Can you work these out from the model? Positions are in its coordinate system, mm. Face numbers are marked on the shaded views. A direction names the side the tool comes from. Coordinates: 2 decimals unless noted, no trailing zeros. Loops run counter-clockwise (first coordinate to the right, second up) from the corner with the lowest first, then second, coordinate; pieces in that order, holes last.
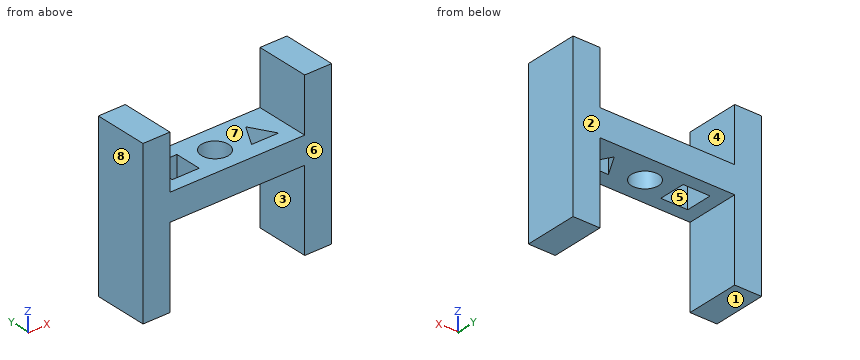
```python
from build123d import *

# Parameters (mm, degrees)
F1_DEPTH = 25.4
F2_W     = 12.7
F2_H     = 12.7
F3_DEPTH = 25.4
F4_R     = 6.35
F5_DEPTH = 25.4
F7_DEPTH = 25.4


with BuildPart() as f1:
    # F0 (on Front) → F1 (new body)
    with BuildSketch(Plane.XZ):
        Polygon((-46.628909, 38.1), (-59.328909, 38.1), (-59.328909, -38.1), (-46.628909, -38.1), (-46.628909, 0), (16.871091, 0), (16.871091, -38.1), (29.571091, -38.1), (29.571091, 38.1), (16.871091, 38.1), (16.871091, 12.7), (-46.628909, 12.7), align=None)
    extrude(amount=F1_DEPTH)

    # F2 (on face) → F3 (cut)
    with BuildSketch(Plane.XY.offset(12.7)):
        with Locations((-33.928909, -12.7)):
            Rectangle(F2_W, F2_H)
    extrude(amount=-F3_DEPTH, mode=Mode.SUBTRACT)

    # F4 (on face) → F5 (cut)
    with BuildSketch(Plane.XY.offset(12.7)):
        with Locations((-14.878909, -12.7)):
            Circle(F4_R)
    extrude(amount=-F5_DEPTH, mode=Mode.SUBTRACT)

    # F6 (on face) → F7 (cut)
    with BuildSketch(Plane.XY.offset(12.7)):
        Polygon((4.171091, -7.2009), (-2.178909, -18.199423), (10.521091, -18.199423), align=None)
    extrude(amount=-F7_DEPTH, mode=Mode.SUBTRACT)


solid = f1.part
```
Item 1: We'd pull the mould along X, two halves only. Please class the marked faces 6, 7 and 8: +X half, -X half, draft (parallel to the pull), parting line (faces both ways), or undercut.
Results are:
face 6: draft
face 7: undercut
face 8: -X half
Item 2: Suppose I cut it at B-B, the plane z = 14. Please give me the cut outline in (x, y), plus the area to 3 significant figures.
Results are:
outline: (-59.33, -25.4) - (-46.63, -25.4) - (-46.63, 0) - (-59.33, 0) - close; (16.87, -25.4) - (29.57, -25.4) - (29.57, 0) - (16.87, 0) - close
area: 645 mm2
Item 3: Suppose I cut it at C-C, the plane y = -22. Please give me the cut outline in (x, z).
Results are:
outline: (-59.33, -38.1) - (-46.63, -38.1) - (-46.63, 0) - (16.87, 0) - (16.87, -38.1) - (29.57, -38.1) - (29.57, 38.1) - (16.87, 38.1) - (16.87, 12.7) - (-46.63, 12.7) - (-46.63, 38.1) - (-59.33, 38.1) - close
Item 4: Suppose I cut it at A-A, the plane x = -35.5. Please give me the cut outline in (y, z), plus the area to 3 significant figures.
Results are:
outline: (-25.4, 0) - (-19.05, 0) - (-19.05, 12.7) - (-25.4, 12.7) - close; (-6.35, 0) - (0, 0) - (0, 12.7) - (-6.35, 12.7) - close
area: 161 mm2
Item 5: I'm going to push flat-ended pins straight in: P1, Ø12.5, axis at x = -21.5, y = -17.5, coming from the +Z side; P2, Ø10, axis at x = 10, z = -8, coming from the -Y side. Where does each tip first touch, or does it pass through?
Results are:
P1: stops at z = 12.7
P2: passes through
Item 6: On a 3-axis mill with a long thin cutter (end or side, diameter ignored), from which of +Z, -Z, +X, -X, +Y, -Y can I reach the whole of each face in a straight line? I mean the marked faces 1, 2, 3, 4 and 5. Say none if no direction works.
Results are:
face 1: -Z, +X, -X, +Y, -Y
face 2: +Z, -Z, +X, -X, +Y
face 3: -Z, +Y, -Y
face 4: +Z, +Y, -Y
face 5: +Z, -Z
Item 7: I need wall thicknesses on line 1 along X through (y, z) = (-3.75, -32.5); line 2 along X through (y, z) = (-17.5, 6.5); line 3 along X through (y, z) = (-10, 6.5). Which ranges of each line are inside material? Lowest first, please.
Results are:
line 1: x = -59.33 to -46.63, 16.87 to 29.57
line 2: x = -59.33 to -40.28, -27.58 to -19.04, -10.72 to -1.78, 10.12 to 29.57
line 3: x = -59.33 to -40.28, -27.58 to -20.63, -9.13 to 2.56, 5.79 to 29.57
Item 8: Suppose I cut it at D-D, the plane y = -12.7. Please give me the cut outline in (x, z).
Results are:
outline: (-59.33, -38.1) - (-46.63, -38.1) - (-46.63, 0) - (-40.28, 0) - (-40.28, 12.7) - (-46.63, 12.7) - (-46.63, 38.1) - (-59.33, 38.1) - close; (-27.58, 0) - (-21.23, 0) - (-21.23, 12.7) - (-27.58, 12.7) - close; (-8.53, 0) - (1, 0) - (1, 12.7) - (-8.53, 12.7) - close; (7.35, 0) - (16.87, 0) - (16.87, -38.1) - (29.57, -38.1) - (29.57, 38.1) - (16.87, 38.1) - (16.87, 12.7) - (7.35, 12.7) - close
